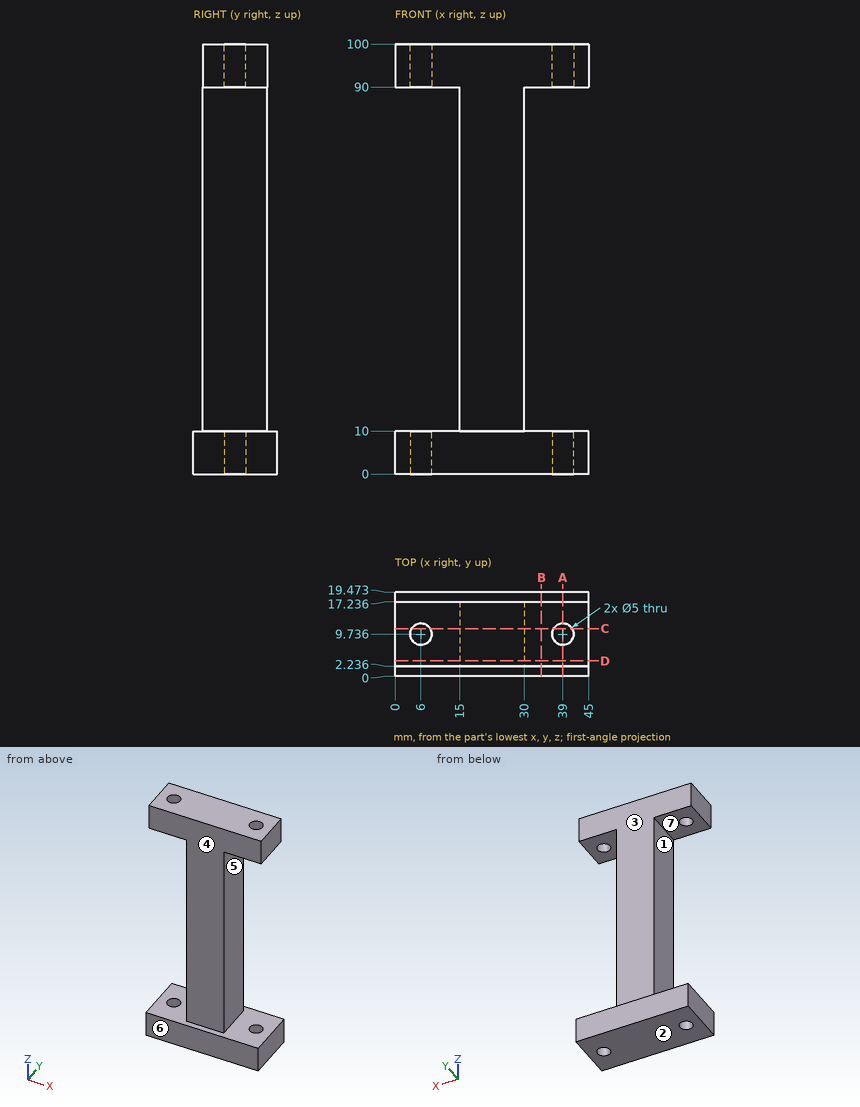
Geometry: see drawing. Coordinates: mm, zero at the bounding-box minimum. A direction names the side the tool comes from. Round coordinates to 2 decimals unless told otherwise and drop trailing zeros. Loops run counter-clockwise (first coordinate to the right, second up) from the corner with the lowest first, then second, coordinate; pieces in that order, holes last. Notation, with made-up numbers: (8.25, -38) -> (65.25, -38) arc R17 ccw to (65.25, -13) -> close; hole circle Ø10 at (11.5, 26). An arc over 180 degrees is marked (long way). Write each question's results on one line, items separated by ' | '.
Item 1: Cut plane C-C on y = 11. Return the cut outline in (x, z), and give its area (3 significant figures).
Answers below:
outline: (0, 0) -> (3.84, 0) -> (3.84, 10) -> (0, 10) -> close; (0, 90) -> (3.84, 90) -> (3.84, 100) -> (0, 100) -> close; (8.16, 0) -> (36.84, 0) -> (36.84, 10) -> (30, 10) -> (30, 90) -> (36.84, 90) -> (36.84, 100) -> (8.16, 100) -> (8.16, 90) -> (15, 90) -> (15, 10) -> (8.16, 10) -> close; (41.16, 0) -> (45, 0) -> (45, 10) -> (41.16, 10) -> close; (41.16, 90) -> (45, 90) -> (45, 100) -> (41.16, 100) -> close | area: 1,930 mm²
Item 2: Set-up query: the marked faces 4, 5, 6 and 7. Return all of +Z, -Z, +X, -X, +Y, -Y with unobstructed straight access to the full face (end or side cutting, diameter ignored); none if empty.
Answers below:
face 4: +Z, +X, -X, -Y | face 5: +X, +Y, -Y | face 6: +Z, -Z, +X, -X, -Y | face 7: -X, +Y, -Y
Item 3: Pin query (flat end, axial travel): pin 1 Ø4.5 at (y, z) = (11.5, 69.5) entering from -X; pin 2 Ø6 at (x, y) = (39, 9.74) entering from -Z; pin 3 Ø2 at (x, z) = (25, 47) entering from -Y; pin 4 Ø13.5 at (x, z) = (12.5, 62.5) entering from +Y. Return the tip coordinate at first contact, or that it passes through.
Answers below:
pin 1: stops at x = 15 | pin 2: stops at z = 0 | pin 3: stops at y = 2.24 | pin 4: stops at y = 17.24
Item 4: Cut plane D-D on y = 3.5. Return the cut outline in (x, z).
Answers below:
outline: (0, 0) -> (45, 0) -> (45, 10) -> (30, 10) -> (30, 90) -> (45, 90) -> (45, 100) -> (0, 100) -> (0, 90) -> (15, 90) -> (15, 10) -> (0, 10) -> close
Item 5: Pull-direction query (Z, two-part tool) for the marked faces 1, 2 and 3; classes: pulls with the +Z half, pulls with the -Z half, needs draft (parallel to the pull), parting line crosses it, or undercut.
Answers below:
face 1: undercut | face 2: pulls with the -Z half | face 3: needs draft
Item 6: Line query: probe 1 along Z at (x, y) = (35, 12); probe 2 along Y at (x, z) = (39, 7); probe 3 along X at (y, z) = (16.75, 88). Output: solid intervals per line, ascending. Write a range as [from, to].
Answers below:
probe 1: z = [0, 10], [90, 100] | probe 2: y = [0, 7.24], [12.24, 19.47] | probe 3: x = [15, 30]
Item 7: Cut plane A-A on x = 39. Return the cut outline in (y, z).
Answers below:
outline: (0, 0) -> (7.24, 0) -> (7.24, 10) -> (0, 10) -> close; (2.24, 90) -> (7.24, 90) -> (7.24, 100) -> (2.24, 100) -> close; (12.24, 0) -> (19.47, 0) -> (19.47, 10) -> (12.24, 10) -> close; (12.24, 90) -> (17.24, 90) -> (17.24, 100) -> (12.24, 100) -> close
Item 8: Cut plane B-B on x = 34. Return the cut outline in (y, z), and give its area (3 significant figures).
Answers below:
outline: (0, 0) -> (19.47, 0) -> (19.47, 10) -> (0, 10) -> close; (2.24, 90) -> (17.24, 90) -> (17.24, 100) -> (2.24, 100) -> close | area: 345 mm²
